```python
from build123d import *

# Parameters (mm, degrees)
SKETCH1_W           = 22
SKETCH1_H           = 22
BOSS_EXTRUDE1_DEPTH = 2
SKETCH2_R           = 7.35
BOSS_EXTRUDE2_DEPTH = 4
SKETCH3_R           = 2.5
BOSS_EXTRUDE3_DEPTH = 3
SKETCH4_R           = 1.6
CUT_EXTRUDE1_DEPTH  = 17.340134638
CIRPATTERN1_COUNT   = 4
FILLET1_R           = 2.5


with BuildPart() as part:
    # Sketch1 → Boss-Extrude1 (new body)
    with BuildSketch(Plane(origin=(0, 0, 0), x_dir=(1, 0, 0), z_dir=(0, 1, 0))):
        Rectangle(SKETCH1_W, SKETCH1_H)
    extrude(amount=BOSS_EXTRUDE1_DEPTH)

    # Sketch2 → Boss-Extrude2 (add)
    with BuildSketch(Plane(origin=(0, 2, 0), x_dir=(1, 0, 0), z_dir=(0, 1, 0))):
        with Locations(Location((0, 0, 0), (0, 0, 270))):
            Circle(SKETCH2_R)
    extrude(amount=BOSS_EXTRUDE2_DEPTH)

    # Sketch3 → Boss-Extrude3 (add)
    with BuildSketch(Plane(origin=(0, 2, 0), x_dir=(1, 0, 0), z_dir=(0, 1, 0))):
        with Locations(Location((-8.5, -8.5, 0), (0, 0, 270))):
            Circle(SKETCH3_R)
    boss_extrude3 = extrude(amount=BOSS_EXTRUDE3_DEPTH)

    # Sketch4 → Cut-Extrude1 (cut, through all)
    with BuildSketch(Plane(origin=(0, 5, 0), x_dir=(1, 0, 0), z_dir=(0, 1, 0))):
        with Locations(Location((-8.5, -8.5, 0), (0, 0, 270))):
            Circle(SKETCH4_R)
    cut_extrude1 = extrude(amount=-CUT_EXTRUDE1_DEPTH, mode=Mode.SUBTRACT)

    # CirPattern1: Boss-Extrude3, Cut-Extrude1 ×4 about axis
    cirpattern1_axis = Axis((0, 0, 0), (0, 1, 0))
    add([boss_extrude3.rotate(cirpattern1_axis, i * 360 / CIRPATTERN1_COUNT) for i in range(1, CIRPATTERN1_COUNT)])
    add([cut_extrude1.rotate(cirpattern1_axis, i * 360 / CIRPATTERN1_COUNT) for i in range(1, CIRPATTERN1_COUNT)], mode=Mode.SUBTRACT)

    # Fillet1
    fillet1_edges = [part.edges().sort_by_distance(p)[0] for p in [
        (11, 1, -11),
        (-11, 1, -11),
        (11, 1, 11),
        (-11, 1, 11),
    ]]
    fillet(fillet1_edges, radius=FILLET1_R - 0.0001)  # a hair under: the kernel refuses the full size


solid = part.part
```
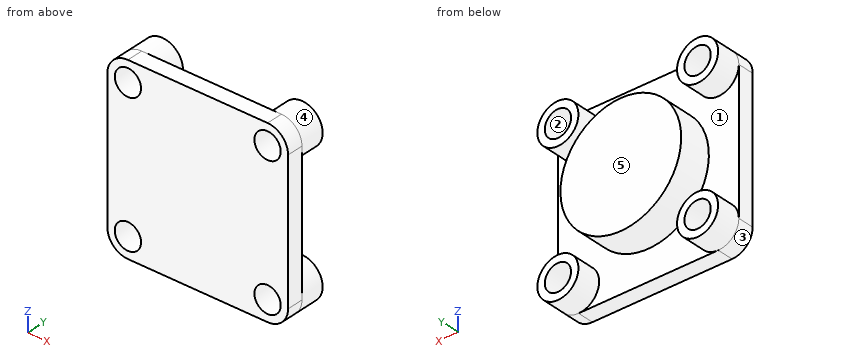
Here's how the part is built. I have some questions about the finished solid (model axes, mm). Face numbers are marked on the shaded views. A direction names the side the tool comes from. Coordinates: 2 decimals unless noted, no trailing zeros. Write each loop counter-clockwise with the first axis right and the second up, starting at its lowest first coordinate (ties: lowest second). Pieces come first, ordered by that corner, then holes. Notation, with made-up numbers: (40, -6.75) - (58, -6.75) arc R10 cw to (58, 3.25) - close; hole circle Ø9 at (-26.5, 30). An arc over 180 degrees is marked (long way). One line per item, written item: value.
1) We'd pull the mould along X, two halves only. Please class the marked faces 3, 4 and 5: pulls with the +X half, pulls with the -X half, needs draft (parallel to the pull), parting line crosses it, or undercut.
Model answer:
face 3: pulls with the -X half
face 4: undercut
face 5: needs draft
2) I need wall thicknesses on line 1 along Y through (x, z) = (7, -5.5); line 2 along X through (y, z) = (2.85, -9.5). Which ranges of each line are inside material? Lowest first, please.
Model answer:
line 1: y = 0 to 2
line 2: x = -10.79 to -9.75, -7.25 to -6.21, 6.21 to 7.25, 9.75 to 10.79
3) Suppose I cut it at D-D on z = 0. Write out the boundary of the cut face in (x, y), and give its area (3 significant figures).
Model answer:
outline: (-11, 0) - (11, 0) - (11, 2) - (7.35, 2) - (7.35, 6) - (-7.35, 6) - (-7.35, 2) - (-11, 2) - close
area: 103 mm²
4) On a 3-axis mill with a long thin cutter (end or side, diameter ignored), from which of +Z, -Z, +X, -X, +Y, -Y can I reach the whole of each face in a straight line? I mean the marked faces 1 and 2. Say none if no direction works.
Model answer:
face 1: +Y
face 2: +Y, -Y
5) Suppose I cut it at A-A on y = 4.15. State how many separate pieces and enclosed holes the cut face has, and give its area (3 significant figures).
Model answer:
separate pieces: 5
enclosed holes: 4
area: 216 mm²
6) Suppose I cut it at B-B on y = 0.55. Write out the boundary of the cut face in (x, z), and give its area (3 significant figures).
Model answer:
outline: (-11, -8.5) arc R2.5 ccw to (-8.5, -11) - (8.5, -11) arc R2.5 ccw to (11, -8.5) - (11, 8.5) arc R2.5 ccw to (8.5, 11) - (-8.5, 11) arc R2.5 ccw to (-11, 8.5) - close; hole circle Ø3.2 at (-8.5, -8.5); hole circle Ø3.2 at (-8.5, 8.5); hole circle Ø3.2 at (8.5, -8.5); hole circle Ø3.2 at (8.5, 8.5)
area: 446 mm²
7) Suppose I cut it at C-C on x = 0. Write out the boundary of the cut face in (y, z), and give its area (3 significant figures).
Model answer:
outline: (0, -11) - (2, -11) - (2, -7.35) - (6, -7.35) - (6, 7.35) - (2, 7.35) - (2, 11) - (0, 11) - close
area: 103 mm²
8) I'm going to push flat-ended pins straight in: P1, Ø1.5, axis at y = 3.5, z = -2.5, coming from the +X side; P2, Ø2.5, axis at x = 9.5, z = -9, coming from the +Y side; P3, Ø1.5, axis at x = -5.5, y = 5, coming from the -Z side. Where does each tip first touch, or does it pass through?
Model answer:
P1: stops at x = 7.14
P2: stops at y = 5
P3: stops at z = -9.59
